Verification items for the finished model (mm, model axes). A direction names the side the tool comes from. Give positions to 0.01 mm unless a question says otherwise; leave off trailing zeros. Loops run counter-clockwise (first coordinate to the right, second up) from the corner with the lowest first, then second, coordinate; pieces in that order, holes last. Notation, with made-up numbers: (62, -11) -> (71, -11) arc R14 ccw to (71, -4) -> close; hole circle Ø5 at (34, 71). An arc over 180 degrees is marked (long way). Use one line per item in the form item = value. Start each with the question number.
from build123d import *

# Parameters (mm, degrees)
SKETCH3_R           = 22
BOSS_EXTRUDE1_DEPTH = 70
SKETCH14_W          = 80
SKETCH14_H          = 20
BOSS_EXTRUDE3_DEPTH = 10
SKETCH4_R           = 19
CUT_EXTRUDE1_DEPTH  = 65
SKETCH5_R           = 3.5
CUT_EXTRUDE2_DEPTH  = 5
SKETCH7_R           = 1.5
CUT_EXTRUDE3_DEPTH  = 5
SKETCH15_R          = 2
CUT_EXTRUDE6_DEPTH  = 10
FILLET1_R           = 10
FILLET2_R           = 10
FILLET3_R           = 10
FILLET4_R           = 1
SKETCH16_R          = 11
CUT_EXTRUDE7_DEPTH  = 2


with BuildPart() as part:
    # Sketch3 → Boss-Extrude1 (new body)
    with BuildSketch(Plane(origin=(0, 0, 0), x_dir=(1, 0, 0), z_dir=(0, 1, 0))):
        with Locations(Location((0, 0, 0), (0, 0, 270))):
            Circle(SKETCH3_R)
    extrude(amount=BOSS_EXTRUDE1_DEPTH)

    # Sketch14 → Boss-Extrude3 (add)
    with BuildSketch(Plane(origin=(0, 70, 0), x_dir=(1, 0, 0), z_dir=(0, 1, 0))):
        Rectangle(SKETCH14_W, SKETCH14_H)
    extrude(amount=-BOSS_EXTRUDE3_DEPTH)

    # Sketch4 → Cut-Extrude1 (cut)
    with BuildSketch(Plane(origin=(0, 0, 0), x_dir=(-1, 0, 0), z_dir=(0, -1, 0))):
        with Locations(Location((0, 0, 0), (0, 0, 90))):
            Circle(SKETCH4_R)
    extrude(amount=-CUT_EXTRUDE1_DEPTH, mode=Mode.SUBTRACT)

    # Sketch5 → Cut-Extrude2 (cut)
    with BuildSketch(Plane(origin=(0, 70, 0), x_dir=(1, 0, 0), z_dir=(0, 1, 0))):
        with Locations(Location((0, 0, 0), (0, 0, 270))):
            Circle(SKETCH5_R)
    extrude(amount=-CUT_EXTRUDE2_DEPTH, mode=Mode.SUBTRACT)

    # Sketch7 → Cut-Extrude3 (cut)
    with BuildSketch(Plane(origin=(0, 70, 0), x_dir=(1, 0, 0), z_dir=(0, 1, 0))):
        with Locations(Location((0, -14, 0), (0, 0, 270))):
            Circle(SKETCH7_R)
        with Locations(Location((0, 14, 0), (0, 0, 270))):
            Circle(SKETCH7_R)
        with Locations(Location((14, 0, 0), (0, 0, 270))):
            Circle(SKETCH7_R)
        with Locations(Location((-14, 0, 0), (0, 0, 270))):
            Circle(SKETCH7_R)
    extrude(amount=-CUT_EXTRUDE3_DEPTH, mode=Mode.SUBTRACT)

    # Sketch15 → Cut-Extrude6 (cut)
    with BuildSketch(Plane(origin=(0, 70, 0), x_dir=(1, 0, 0), z_dir=(0, 1, 0))):
        with Locations(Location((30, 0, 0), (0, 0, 270))):
            Circle(SKETCH15_R)
        with Locations(Location((-30, 0, 0), (0, 0, 270))):
            Circle(SKETCH15_R)
    extrude(amount=-CUT_EXTRUDE6_DEPTH, mode=Mode.SUBTRACT)

    # Fillet1
    fillet1_edges = [part.edges().sort_by_distance(p)[0] for p in [
        (40, 65, -10),
        (40, 65, 10),
    ]]
    fillet(fillet1_edges, radius=FILLET1_R - 0.0001)  # a hair under: the kernel refuses the full size

    # Fillet2
    fillet2_edges = [part.edges().sort_by_distance(p)[0] for p in [
        (-40, 65, -10),
        (-40, 65, 10),
    ]]
    fillet(fillet2_edges, radius=FILLET2_R - 0.0001)  # a hair under: the kernel refuses the full size

    # Fillet3
    fillet3_edges = [part.edges().sort_by_distance(p)[0] for p in [
        (-19.595917942, 65, 10),
        (19.595917942, 65, 10),
        (19.595917942, 65, -10),
        (-19.595917942, 65, -10),
    ]]
    fillet(fillet3_edges, radius=FILLET3_R)

    # Fillet4
    fillet4_edges = [part.edges().sort_by_distance(p)[0] for p in [
        (0, 0, -22),
        (0, 0, 19),
    ]]
    fillet(fillet4_edges, radius=FILLET4_R)

    # Sketch16 → Cut-Extrude7 (cut)
    with BuildSketch(Plane.XZ.offset(-65)):
        with Locations(Location((0, 0, 0), (0, 0, 270))):
            Circle(SKETCH16_R)
    extrude(amount=-CUT_EXTRUDE7_DEPTH, mode=Mode.SUBTRACT)


solid = part.part
Item 1: Material ranges on line 1 (X direction, y = 65.25, z = 0); line 2 (X direction, y = 68.9, z = 0); line 3 (X direction, y = 64.75, z = 0), recorded low to high.
Item 2: Gauge pin test, flat ends, axial feed: pin 1 Ø4.5 at (x, z) = (30, 0) entering from -Y; pin 2 Ø17.5 at (x, z) = (2, 4.5) entering from -Y; pin 3 Ø1.5 at (x, y) = (19.5, 15) entering from -Z; pin 4 Ø2.5 at (x, z) = (0, -14) entering from -Y (3 decimals). Record the tip position at first contact, or that the pin passes through.
Item 3: Sectioned sample at B-B, the plane y = 53.5. Enter the section's corners in (x, z).
Item 4: Sectioned sample at C-C, the plane x = 33.5. Enter the section's corners in (y, z), and give its area (3 significant figures).
Item 5: Sectioned sample at A-A, the plane x = 0. Enter the section's corners in (y, z), and give its area (3 significant figures).
Item 6: Draft check along Z on faces 1 (the cylindrical face through (-11.56, 32.55, 15.08)), 2 (the cylindrical face through (14.45, 67.54, 1.43)), 3 (the flat face through (27, 65, 10)), 4 (the cylindrical face through (36.99, 64.93, -7.15)). Enter one of: +Z half, -Z half, draft (parallel to the pull), parting line (faces both ways), or undercut.
Item 7: Tool access check on faces 5 (the flat face through (-28, 65, 10)), 6 (the flat face through (3, 67, 3)), 7 (the flat face through (-8, 0, 19)), 8 (the flat face through (-28, 65, -10)). Record the directions out of +Z, -Z, +X, -X, +Y, -Y that give a thin tool (end or side, any length) a straight path to the whole face; none if there is none.
Outcome:
q1.line_1 = -40 to -32, -28 to -15.5, -12.5 to -11, 11 to 12.5, 15.5 to 28, 32 to 40
q1.line_2 = -40 to -32, -28 to -15.5, -12.5 to -3.5, 3.5 to 12.5, 15.5 to 28, 32 to 40
q1.line_3 = -40 to -32, -28 to -19, 19 to 28, 32 to 40
q2.pin_1 = 60
q2.pin_2 = 65
q2.pin_3 = -11.51
q2.pin_4 = through
q3.outline = circle Ø44 at (0, 0); hole circle Ø38 at (0, 0)
q4.outline = (60, -9.37) -> (70, -9.37) -> (70, 9.37) -> (60, 9.37) -> close
q4.area = 187 mm^2
q5.outline = (0, -21) arc R1 ccw to (1, -22) -> (70, -22) -> (70, -15.5) -> (65, -15.5) -> (65, -19) -> (1, -19) arc R1 ccw to (0, -20) -> close; (0, 20) arc R1 ccw to (1, 19) -> (65, 19) -> (65, 15.5) -> (70, 15.5) -> (70, 22) -> (1, 22) arc R1 ccw to (0, 21) -> close; (65, -12.5) -> (70, -12.5) -> (70, -3.5) -> (67, -3.5) -> (67, -11) -> (65, -11) -> close; (65, 11) -> (67, 11) -> (67, 3.5) -> (70, 3.5) -> (70, 12.5) -> (65, 12.5) -> close
q5.area = 514 mm^2
q6.face_1 = undercut
q6.face_2 = undercut
q6.face_3 = +Z half
q6.face_4 = -Z half
q7.face_5 = +Z, -X, +Y, -Y
q7.face_6 = -Y
q7.face_7 = +Z, -Z, +X, -X, -Y
q7.face_8 = -Z, -X, +Y, -Y
